Here's how the part is built. I have some questions about the finished solid (model axes, mm). Face numbers are marked on the shaded views. Give positions to 0.01 mm unless a question says otherwise; leave off trailing zeros. Loops run counter-clockwise (first coordinate to the right, second up) from the corner with the lowest first, then second, coordinate; pieces in that order, holes last. Notation, with made-up numbers: M 15,2 L 40,2 A6 cw 40,13 Z; hole C -29,46.25 d1. An arc over 180 degrees is marked long. Answer as CSV lines item,"result". Start each with the question number.
Item 1: I want a section at C-C on y = 11.5. List the corners of the cut face in (x, z) for me, plus the area to 3 significant figures.
Item 2: I want a section at B-B on x = 48. List the corners of the cut face in (y, z) for me, plus the area to 3 significant figures.
Item 3: I want a section at D-D on x = -42. List the corners of the cut face in (y, z) for me.
Item 4: If I drill on line 1 along Z through (x, y) = (-1, 4.75); line 2 along Z through (x, y) = (37, 2.25); line 3 along Z through (x, y) = (25.5, 2.25), over which ranges is the centre line in solid material (lowest first)? Write a range as from..to.
Item 5: I want a section at A-A on z = -3. List the corners of the cut face in (x, y) for me.
Item 6: Will these pins go through, and if not, where does the flat tip stop? P1, Ø3, axis at x = 15.5, z = 40, coming from the +Y side; P2, Ø4.5, axis at x = 29.48, z = 10.83, coming from the +Y side; P3, Ø2, axis at x = -26, z = -77.5, coming from the +Y side.
Item 7: If we mould it in two halves opening along X, with no side actions, what happens to the marked faces 1 and 2? For each: released by +X, released by -X, zero draft, split by the parting line, or undercut.
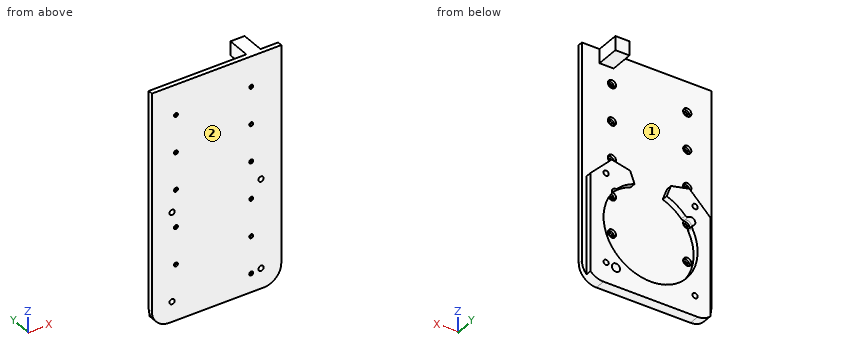
from build123d import *

# Parameters (mm, degrees)
ESQUISSE1_W                                        = 110.05441198
ESQUISSE1_H                                        = 4
BOSS_EXTRU_1_DEPTH                                 = 100
CHAMBRAGE_POUR_VIS_T_TE_RONDE_BOMB_E_M_D           = 3.4
CHAMBRAGE_POUR_VIS_T_TE_RONDE_BOMB_E_M_CBORE_D     = 7
CHAMBRAGE_POUR_VIS_T_TE_RONDE_BOMB_E_M_CBORE_DEPTH = 2.4
BOSS_EXTRU_2_START                                 = 5
ESQUISSE2_R                                        = 3.5
BOSS_EXTRU_2_DEPTH                                 = 5
CONG_1_R                                           = 15
DIAM_TRE_DU_PER_AGE_4_5_4_5_1_D                    = 4.5
R_P_TITION_CIRCULAIRE1_COUNT                       = 4
CONG_2_R                                           = 2
ESQUISSE12_W                                       = 12
ESQUISSE12_H                                       = 12
BOSS_EXTRU_3_DEPTH                                 = 20


with BuildPart() as part:
    # Esquisse1 → Boss.-Extru.1 (new, symmetric)
    with BuildSketch(Plane.XY):
        with Locations((0, -2)):
            Rectangle(ESQUISSE1_W, ESQUISSE1_H)
    extrude(amount=BOSS_EXTRU_1_DEPTH, both=True)

    # Chambrage pour vis à tête ronde bombée M31 (through all)
    with Locations(Plane(origin=(0, 0, 0), x_dir=(-1, 0, 0), z_dir=(0, 1, 0))):
        with Locations((-29.475226789, 74.166108561), (-29.475226789, 42.499553515), (-29.475226789, 10.83299847), (-29.475226789, -20.833556576), (-29.475226789, -52.500111621), (-29.475226789, -84.166666667), (34.58023462, -52.500111621), (34.58023462, -20.833556576), (34.58023462, 10.83299847), (34.58023462, 42.499553515), (34.58023462, 74.166108561)):
            CounterBoreHole(CHAMBRAGE_POUR_VIS_T_TE_RONDE_BOMB_E_M_D / 2, CHAMBRAGE_POUR_VIS_T_TE_RONDE_BOMB_E_M_CBORE_D / 2, CHAMBRAGE_POUR_VIS_T_TE_RONDE_BOMB_E_M_CBORE_DEPTH)

    # Esquisse2 → Boss.-Extru.2 (add)
    with BuildSketch(Plane(origin=(0, 0, 0), x_dir=(1, 0, 0), z_dir=(0, 1, 0)).offset(BOSS_EXTRU_2_START)):
        with BuildLine():
            ThreePointArc((-34.266288353, 24.319447816), (-30.921403648, 70.407647487), (13.653919587, 82.587588418))
            ThreePointArc((13.653919587, 82.587588418), (28.258676617, 73.282659801), (37.561941061, 58.676842631))
            ThreePointArc((37.561941061, 58.676842631), (39.631466487, 39.785625854), (32.749013114, 22.071426963))
            ThreePointArc((32.749013114, 22.071426963), (32.18281347, 18.615680482), (28.906205557, 17.380121353))
            ThreePointArc((28.906205557, 17.380121353), (21.853265177, 11.515003633), (13.649636645, 7.410852954))
            Line((13.649636645, 7.410852954), (17.29324483, -2.597524835))
            Line((17.29324483, -2.597524835), (33.030412308, -6.085123148))
            Line((33.030412308, -6.085123148), (51.056358534, 11.938098766))
            Line((51.056358534, 11.938098766), (51.056358534, 100))
            Line((51.056358534, 100), (-51.112329133, 100))
            Line((-51.112329133, 100), (-51.112329133, 11.942381707))
            Line((-51.112329133, 11.942381707), (-33.08910722, -6.083564519))
            Line((-33.08910722, -6.083564519), (-17.351939742, -2.595966207))
            Line((-17.351939742, -2.595966207), (-13.708331558, 7.412411582))
            ThreePointArc((-13.708331558, 7.412411582), (-23.310602668, 12.474879878), (-31.198165181, 19.932664624))
            ThreePointArc((-31.198165181, 19.932664624), (-37.448352421, 18.827590404), (-34.266288353, 24.319447816))
        make_face()
        with Locations(Location((29.475226789, 84.166666667, 0), (0, 0, 269.999999999))):
            Circle(ESQUISSE2_R, mode=Mode.SUBTRACT)
    extrude(amount=-BOSS_EXTRU_2_DEPTH)

    # Congé1
    cong_1_edges = [part.edges().sort_by_distance(p)[0] for p in [
        (55.02720599, -2, -100),
        (-55.02720599, -2, -100),
    ]]
    fillet(cong_1_edges, radius=CONG_1_R)

    # Diamètre du perçage Ø4.5 (4.5)1 (through all)
    with Locations(Plane(origin=(0, 5, 0), x_dir=(1, 0, 0), z_dir=(0, 1, 0))):
        with Locations((37.80586561, 7.172646225)):
            diam_tre_du_per_age_4_5_4_5_1 = Hole(DIAM_TRE_DU_PER_AGE_4_5_4_5_1_D / 2)

    # Répétition circulaire1: Diamètre du perçage Ø4.5 (4.5)1 ×4 about axis
    r_p_tition_circulaire1_axis = Axis((-0.027205985, 0, -45), (0, 1, 0))
    for i in range(1, R_P_TITION_CIRCULAIRE1_COUNT):
        add(diam_tre_du_per_age_4_5_4_5_1.rotate(r_p_tition_circulaire1_axis, i * 360 / R_P_TITION_CIRCULAIRE1_COUNT), mode=Mode.SUBTRACT)

    # Congé2
    cong_2_edges = [part.edges().sort_by_distance(p)[0] for p in [
        (-34.266288353, 2.5, -24.319447816),
        (28.906205557, 2.5, -17.380121353),
        (-31.198165181, 2.5, -19.932664624),
    ]]
    fillet(cong_2_edges, radius=CONG_2_R)

    # Esquisse12 → Boss.-Extru.3 (add)
    with BuildSketch(Plane(origin=(0, 0, 0), x_dir=(1, 0, 0), z_dir=(0, 1, 0))):
        with Locations((34.02720599, -94)):
            Rectangle(ESQUISSE12_W, ESQUISSE12_H)
    extrude(amount=BOSS_EXTRU_3_DEPTH)


solid = part.part
Result:
1,outline,"M 28.03,88 L 40.03,88 L 40.03,100 L 28.03,100 Z"
1,area,"144 mm^2"
2,outline,"M -4,-97.71 L 5,-97.71 L 5,-8.88 L 0,-8.88 L 0,100 L -4,100 Z"
2,area,"1,230 mm^2"
3,outline,"M -4,-99.87 L 5,-99.87 L 5,-2.83 L 0,-2.83 L 0,100 L -4,100 Z"
4,line 1,"-100..-84.99"
4,line 2,"-100..-84.94, -80.73..-60.13, -29.87..-9.27, -5.07..2.12, 88..100"
4,line 3,"-100..-75.8, -14.2..4.42"
5,outline,"M -55.03,-4 L 55.03,-4 L 55.03,0 L 42.12,0 L 42.12,5 L 15.26,5 L 15.26,0 L -15.31,0 L -15.31,5 L -42.17,5 L -42.17,0 L -55.03,0 Z"
6,P1,"y = 0"
6,P2,"y = -2.4"
6,P3,"y = 5"
7,face 1,"undercut"
7,face 2,"zero draft"
